Build history of the part. All positions in model axes, mm. A direction names the side the tool comes from. Round coordinates to 2 decimals unless told otherwise and drop trailing zeros. Write each loop counter-clockwise with the first axis right and the second up, starting at its lowest first coordinate (ties: lowest second). Pieces come first, ordered by that corner, then holes. Notation, with made-up numbers: M 52.25,62.5 L 60.25,62.5 A25 cw 60.25,84.5 Z; hole C 16,-4.75 d10. An arc over 180 degrees is marked long. One line per item, written item: value. Start each with the question number.
```python
from build123d import *

# Parameters (mm, degrees)
F1_DEPTH = 50.8
F3_DEPTH = 50.8
F4_R     = 2.54
F5_R     = 2.54
F6_R     = 2.54
F8_DEPTH = 50.8


with BuildPart() as f1:
    # F0 (on Top) → F1 (new body)
    with BuildSketch(Plane.XY):
        with BuildLine():
            ThreePointArc((-111.331622, 89), (-115.642145, 87.214523), (-117.427622, 82.904))
            Line((-117.427622, 82.904), (-117.427622, -82.904))
            ThreePointArc((-117.427622, -82.904), (-115.642145, -87.214523), (-111.331622, -89))
            Line((-111.331622, -89), (111.331622, -89))
            ThreePointArc((111.331622, -89), (115.642145, -87.214523), (117.427622, -82.904))
            Line((117.427622, -82.904), (117.427622, 82.904))
            ThreePointArc((117.427622, 82.904), (115.642145, 87.214523), (111.331622, 89))
            Line((111.331622, 89), (-111.331622, 89))
        make_face()
    extrude(amount=F1_DEPTH)

    # F2 (on face) → F3 (cut)
    with BuildSketch(Plane.XY.offset(50.8)):
        with BuildLine():
            Line((104.473619, 22.683125), (-104.473626, 22.683125))
            ThreePointArc((-104.473626, 22.683125), (-108.963754, 20.823253), (-110.823626, 16.333125))
            Line((-110.823626, 16.333125), (-110.823626, 4.395125))
            ThreePointArc((-110.823626, 4.395125), (-108.963754, -0.095003), (-104.473626, -1.954875))
            Line((-104.473626, -1.954875), (104.473619, -1.954875))
            ThreePointArc((104.473619, -1.954875), (108.963747, -0.095003), (110.823619, 4.395125))
            Line((110.823619, 4.395125), (110.823619, 16.333125))
            ThreePointArc((110.823619, 16.333125), (108.963747, 20.823253), (104.473619, 22.683125))
        make_face()
        with BuildLine():
            ThreePointArc((-30.480004, -40.517802), (-30.108029, -41.415828), (-29.210004, -41.787802))
            Line((-29.210004, -41.787802), (2.539996, -41.787802))
            Line((2.539996, -41.787802), (22.859996, -41.787802))
            Line((22.859996, -41.787802), (29.209996, -41.787802))
            ThreePointArc((29.209996, -41.787802), (30.108022, -41.415828), (30.479996, -40.517802))
            Line((30.479996, -40.517802), (30.479996, -10.037802))
            ThreePointArc((30.479996, -10.037802), (30.108022, -9.139777), (29.209996, -8.767802))
            Line((29.209996, -8.767802), (-29.210004, -8.767802))
            ThreePointArc((-29.210004, -8.767802), (-30.108029, -9.139777), (-30.480004, -10.037802))
            Line((-30.480004, -10.037802), (-30.480004, -40.517802))
        make_face()
        with BuildLine():
            Line((22.859996, -41.787802), (2.539996, -41.787802))
            Line((2.539996, -41.787802), (2.539996, -48.137802))
            ThreePointArc((2.539996, -48.137802), (2.911971, -49.035828), (3.809996, -49.407802))
            Line((3.809996, -49.407802), (21.589996, -49.407802))
            ThreePointArc((21.589996, -49.407802), (22.488022, -49.035828), (22.859996, -48.137802))
            Line((22.859996, -48.137802), (22.859996, -41.787802))
        make_face()
        with BuildLine():
            ThreePointArc((83.165908, -8.767802), (79.573806, -10.2557), (78.085908, -13.847802))
            Line((78.085908, -13.847802), (78.085908, -46.867802))
            ThreePointArc((78.085908, -46.867802), (79.573806, -50.459905), (83.165908, -51.947802))
            Line((83.165908, -51.947802), (100.945908, -51.947802))
            ThreePointArc((100.945908, -51.947802), (104.538011, -50.459905), (106.025908, -46.867802))
            Line((106.025908, -46.867802), (106.025908, -13.847802))
            ThreePointArc((106.025908, -13.847802), (104.538011, -10.2557), (100.945908, -8.767802))
            Line((100.945908, -8.767802), (83.165908, -8.767802))
        make_face()
        with BuildLine():
            Line((-40.917659, -45.597802), (-40.917659, -10.037802))
            ThreePointArc((-40.917659, -10.037802), (-41.289633, -9.139777), (-42.187659, -8.767802))
            Line((-42.187659, -8.767802), (-48.537659, -8.767802))
            ThreePointArc((-48.537659, -8.767802), (-49.435685, -9.139777), (-49.807659, -10.037802))
            Line((-49.807659, -10.037802), (-49.807659, -45.597802))
            ThreePointArc((-49.807659, -45.597802), (-49.435685, -46.495828), (-48.537659, -46.867802))
            Line((-48.537659, -46.867802), (-42.187659, -46.867802))
            ThreePointArc((-42.187659, -46.867802), (-41.289633, -46.495828), (-40.917659, -45.597802))
        make_face()
        with BuildLine():
            Line((-90.887246, 81.525263), (-106.635246, 81.525263))
            ThreePointArc((-106.635246, 81.525263), (-108.431297, 80.781314), (-109.175246, 78.985263))
            Line((-109.175246, 78.985263), (-109.175246, 46.981263))
            ThreePointArc((-109.175246, 46.981263), (-108.431297, 45.185212), (-106.635246, 44.441263))
            Line((-106.635246, 44.441263), (-90.887246, 44.441263))
            Line((-90.887246, 44.441263), (-90.887246, 81.525263))
        make_face()
        with BuildLine():
            Line((-80.219246, 81.525263), (-90.887246, 81.525263))
            Line((-90.887246, 81.525263), (-90.887246, 44.441263))
            Line((-90.887246, 44.441263), (-90.887246, 33.011263))
            ThreePointArc((-90.887246, 33.011263), (-90.143297, 31.215212), (-88.347246, 30.471263))
            Line((-88.347246, 30.471263), (-54.819246, 30.471263))
            Line((-54.819246, 30.471263), (-54.819246, 43.171263))
            Line((-54.819246, 43.171263), (-54.819246, 78.985263))
            ThreePointArc((-54.819246, 78.985263), (-55.563195, 80.781314), (-57.359246, 81.525263))
            Line((-57.359246, 81.525263), (-65.487246, 81.525263))
            Line((-65.487246, 81.525263), (-65.487246, 71.365263))
            ThreePointArc((-65.487246, 71.365263), (-66.231195, 69.569212), (-68.027246, 68.825263))
            Line((-68.027246, 68.825263), (-77.679246, 68.825263))
            ThreePointArc((-77.679246, 68.825263), (-79.475297, 69.569212), (-80.219246, 71.365263))
            Line((-80.219246, 71.365263), (-80.219246, 81.525263))
        make_face()
        Polygon((-54.819246, 43.171263), (-54.819246, 30.471263), (74.720754, 30.471263), (74.720754, 43.171263), (60.750754, 43.171263), (-40.849246, 43.171263), align=None)
        with BuildLine():
            Line((74.720754, 43.171263), (74.720754, 30.471263))
            Line((74.720754, 30.471263), (82.340754, 30.471263))
            ThreePointArc((82.340754, 30.471263), (84.136805, 31.215212), (84.880754, 33.011263))
            Line((84.880754, 33.011263), (84.880754, 50.233088))
            Line((84.880754, 50.233088), (84.880754, 55.998263))
            Line((84.880754, 55.998263), (84.880754, 61.409088))
            Line((84.880754, 61.409088), (84.880754, 78.985263))
            ThreePointArc((84.880754, 78.985263), (84.136805, 80.781314), (82.340754, 81.525263))
            Line((82.340754, 81.525263), (77.260754, 81.525263))
            ThreePointArc((77.260754, 81.525263), (75.464703, 80.781314), (74.720754, 78.985263))
            Line((74.720754, 78.985263), (74.720754, 43.171263))
        make_face()
        with BuildLine():
            Line((-40.849246, 50.791263), (-40.849246, 43.171263))
            Line((-40.849246, 43.171263), (60.750754, 43.171263))
            Line((60.750754, 43.171263), (60.750754, 50.791263))
            ThreePointArc((60.750754, 50.791263), (60.006805, 52.587314), (58.210754, 53.331263))
            Line((58.210754, 53.331263), (-38.309246, 53.331263))
            ThreePointArc((-38.309246, 53.331263), (-40.105297, 52.587314), (-40.849246, 50.791263))
        make_face()
        with BuildLine():
            Line((84.880754, 55.998263), (84.880754, 50.233088))
            Line((84.880754, 50.233088), (107.740754, 50.233088))
            ThreePointArc((107.740754, 50.233088), (109.536805, 50.977037), (110.280754, 52.773088))
            Line((110.280754, 52.773088), (110.280754, 55.998263))
            Line((110.280754, 55.998263), (84.880754, 55.998263))
        make_face()
        with BuildLine():
            Line((84.880754, 61.409088), (84.880754, 55.998263))
            Line((84.880754, 55.998263), (110.280754, 55.998263))
            Line((110.280754, 55.998263), (110.280754, 58.869088))
            ThreePointArc((110.280754, 58.869088), (109.536805, 60.665139), (107.740754, 61.409088))
            Line((107.740754, 61.409088), (84.880754, 61.409088))
        make_face()
        with BuildLine():
            ThreePointArc((-61.237659, -46.867802), (-60.339633, -46.495828), (-59.967659, -45.597802))
            Line((-59.967659, -45.597802), (-59.967659, -10.037802))
            ThreePointArc((-59.967659, -10.037802), (-60.339633, -9.139777), (-61.237659, -8.767802))
            Line((-61.237659, -8.767802), (-67.587659, -8.767802))
            ThreePointArc((-67.587659, -8.767802), (-68.485685, -9.139777), (-68.857659, -10.037802))
            Line((-68.857659, -10.037802), (-68.857659, -45.597802))
            ThreePointArc((-68.857659, -45.597802), (-68.485685, -46.495828), (-67.587659, -46.867802))
            Line((-67.587659, -46.867802), (-61.237659, -46.867802))
        make_face()
    extrude(amount=-F3_DEPTH, mode=Mode.SUBTRACT)

    # F4
    f4_edges = [f1.edges().sort_by_distance(p)[0] for p in [
        (-54.819246, 43.171263, 25.4),
        (74.720754, 43.171263, 25.4),
        (84.880754, 50.233088, 25.4),
        (84.880754, 61.409088, 25.4),
        (-90.887246, 44.441263, 25.4),
    ]]
    fillet(f4_edges, radius=F4_R)

    # F5
    f5_edges = [f1.edges().sort_by_distance(p)[0] for p in [
        (-40.849246, 43.171263, 25.4),
        (60.750754, 43.171263, 25.4),
    ]]
    fillet(f5_edges, radius=F5_R)

    # F6
    f6_edges = [f1.edges().sort_by_distance(p)[0] for p in [
        (-80.219246, 81.525263, 25.4),
        (-65.487246, 81.525263, 25.4),
    ]]
    fillet(f6_edges, radius=F6_R)

    # F7 (on face) → F8 (cut)
    with BuildSketch(Plane.XY.offset(50.8)):
        with BuildLine():
            Line((25.847686, -67.664004), (-19.557998, -67.664004))
            Line((-19.557998, -67.664004), (-64.963682, -67.664004))
            Line((-64.963682, -67.664004), (-77.977998, -67.664004))
            ThreePointArc((-77.977998, -67.664004), (-81.570101, -66.176106), (-83.057998, -62.584004))
            Line((-83.057998, -62.584004), (-83.057998, -42.264004))
            Line((-83.057998, -42.264004), (-83.057998, -24.546178))
            ThreePointArc((-83.057998, -24.546178), (-84.545896, -20.954076), (-88.137998, -19.466178))
            Line((-88.137998, -19.466178), (-91.947998, -19.466178))
            Line((-91.947998, -19.466178), (-98.231429, -19.466178))
            ThreePointArc((-98.231429, -19.466178), (-99.129455, -19.094204), (-99.501429, -18.196178))
            Line((-99.501429, -18.196178), (-99.501429, -10.547931))
            ThreePointArc((-99.501429, -10.547931), (-99.873404, -9.649905), (-100.771429, -9.277931))
            Line((-100.771429, -9.277931), (-103.377998, -9.277931))
            Line((-103.377998, -9.277931), (-106.552998, -9.277931))
            ThreePointArc((-106.552998, -9.277931), (-107.451024, -9.649905), (-107.822998, -10.547931))
            Line((-107.822998, -10.547931), (-107.822998, -26.591364))
            Line((-107.822998, -26.591364), (-107.822998, -42.623485))
            Line((-107.822998, -42.623485), (-107.822998, -71.474004))
            ThreePointArc((-107.822998, -71.474004), (-104.847203, -78.658208), (-97.662998, -81.634004))
            Line((-97.662998, -81.634004), (-19.557998, -81.634004))
            Line((-19.557998, -81.634004), (58.547002, -81.634004))
            ThreePointArc((58.547002, -81.634004), (65.731206, -78.658208), (68.707002, -71.474004))
            Line((68.707002, -71.474004), (68.707002, -42.623485))
            Line((68.707002, -42.623485), (68.707002, -26.591364))
            Line((68.707002, -26.591364), (68.707002, -10.547931))
            ThreePointArc((68.707002, -10.547931), (68.335027, -9.649905), (67.437002, -9.277931))
            Line((67.437002, -9.277931), (64.262002, -9.277931))
            Line((64.262002, -9.277931), (61.655433, -9.277931))
            ThreePointArc((61.655433, -9.277931), (60.757407, -9.649905), (60.385433, -10.547931))
            Line((60.385433, -10.547931), (60.385433, -18.196178))
            ThreePointArc((60.385433, -18.196178), (60.013458, -19.094204), (59.115433, -19.466178))
            Line((59.115433, -19.466178), (52.832002, -19.466178))
            Line((52.832002, -19.466178), (49.022002, -19.466178))
            ThreePointArc((49.022002, -19.466178), (45.429899, -20.954076), (43.942002, -24.546178))
            Line((43.942002, -24.546178), (43.942002, -42.264004))
            Line((43.942002, -42.264004), (43.942002, -62.584004))
            ThreePointArc((43.942002, -62.584004), (42.454104, -66.176106), (38.862002, -67.664004))
            Line((38.862002, -67.664004), (25.847686, -67.664004))
        make_face()
        with BuildLine():
            Line((-107.822998, -42.623485), (-107.822998, -26.591364))
            ThreePointArc((-107.822998, -26.591364), (-110.597907, -34.607425), (-107.822998, -42.623485))
        make_face()
        with BuildLine():
            ThreePointArc((68.707002, -42.623485), (71.48191, -34.607425), (68.707002, -26.591364))
            Line((68.707002, -26.591364), (68.707002, -42.623485))
        make_face()
    extrude(amount=-F8_DEPTH, mode=Mode.SUBTRACT)


solid = f1.part
```
Item 1: Cut at A-A, the plane y = 75. Write the cut outline in (x, z).
Item 2: Drill centre lines: line 1 (X direction, y = 67.5, z = 48.5); line 2 (X direction, y = 55.5, z = 15.5); line 3 (Y direction, x = 100, z = 8.5). Where is each one in solid material? Low to high.
Item 3: Cut at D-D, the plane z = 22.5. Count the separate pieces of the cut face and the enclosed holes in it, plus the area to 3 significant figures.
Item 4: Cut at B-B, the plane x = 15.5. Write the cut outline in (y, z).
Item 5: Which spindle directions (+Z, -Z, +X, -X, +Y, -Y) get a long thin tool onto all of the face, cutting with end or side? Do faces 5 (the cylindrical face through (79.61, -10.22, 25.76)), 6 (the flat face through (-117.428, 1, 25)). Say none if no direction does.
Item 6: Two-plate mould, pull along Y, no slides. Class faces 1 (the flat face through (-107.823, -57, 26)), 2 (the flat face through (51, -19, 0)), 3 (the flat face through (-2, -89, 25)), 4 (the cylindrical face through (45.47, -20.915, 25.756)): pulls with the +Y half, pulls with the -Y half, needs draft (parallel to the pull), parting line crosses it, or undercut.
Item 7: Cut at C-C, the plane y = 36. Write the cut outline in (x, z).
Computed values:
1. outline: M -117.43,0 L -109.18,0 L -109.18,50.8 L -117.43,50.8 Z; M -80.22,0 L -65.49,0 L -65.49,50.8 L -80.22,50.8 Z; M -54.82,0 L 74.72,0 L 74.72,50.8 L -54.82,50.8 Z; M 84.88,0 L 117.43,0 L 117.43,50.8 L 84.88,50.8 Z
2. line 1: x = -117.43 to -109.18, -54.82 to 74.72, 84.88 to 117.43
2. line 2: x = -117.43 to -109.18, -54.82 to 74.72, 110.28 to 117.43
2. line 3: y = -89 to -51.95, -8.77 to -1.95, 22.68 to 50.23, 61.41 to 89
3. separate pieces: 1
3. enclosed holes: 7
3. area: 21,500 mm2
4. outline: M -89,0 L -81.63,0 L -81.63,50.8 L -89,50.8 Z; M -67.66,0 L -49.41,0 L -49.41,50.8 L -67.66,50.8 Z; M -8.77,0 L -1.95,0 L -1.95,50.8 L -8.77,50.8 Z; M 22.68,0 L 30.47,0 L 30.47,50.8 L 22.68,50.8 Z; M 53.33,0 L 89,0 L 89,50.8 L 53.33,50.8 Z
5. face 5: +Z, -Z
5. face 6: +Z, -Z, -X, +Y, -Y
6. face 1: undercut
6. face 2: needs draft
6. face 3: pulls with the -Y half
6. face 4: undercut
7. outline: M -117.43,0 L -90.89,0 L -90.89,50.8 L -117.43,50.8 Z; M 84.88,0 L 117.43,0 L 117.43,50.8 L 84.88,50.8 Z
